```python
from build123d import *

# Parameters (mm, degrees)
SKETCH1_R          = 158.5
BASE_FLANGE1_DEPTH = 1


# Read off the part's stored shape, not the designer's step: Edge-Flange1
# Sheet-metal steps are written as plain solids
with BuildPart() as part:
    # Sketch1 → Base-Flange1 (new body)
    with BuildSketch(Plane(origin=(0, 0, 0), x_dir=(1, 0, 0), z_dir=(0, 1, 0))):
        with Locations(Location((0, 0, 0), (0, 0, 270))):
            Circle(SKETCH1_R)
    extrude(amount=-BASE_FLANGE1_DEPTH)

    # Edge-Flange1 outline → Edge-Flange1 (revolve)
    with BuildSketch(Plane.XY):
        with BuildLine():
            Line((159.2366, -1.7366), (159.2366, -15))
            Line((159.2366, -15), (160.2366, -15))
            Line((160.2366, -15), (160.2366, -1.7366))
            ThreePointArc((160.2366, -1.7366), (159.727961636, -0.508638364), (158.5, 0))
            Line((158.5, 0), (158.5, -1))
            ThreePointArc((158.5, -1), (159.020854855, -1.215745145), (159.2366, -1.7366))
        make_face()
    revolve(axis=Axis((0, 0, 0), (0, 1, 0)))


solid = part.part
```
Design review of the part built by this model. Coordinates are the model's own, in mm. Give positions to 0.01 mm unless a question says otherwise; leave off trailing zeros. Order: outer loops, then holes, each group sorted by start corner. A loop starts at its lowest first (then second) coordinate and runs counter-clockwise, first axis right, second up. Notation, with made-up numbers: M 62.5,59 L 101.5,59 A29 ccw 101.5,83 Z; hole C -18.75,-37 d8. An arc over 180 degrees is marked long. One line per question, with ' | ' between items. Start each with the question number.
Q1. We need section A-A (x = 0). Write out the cut boundary in (y, z), plus the area to 3 significant figures.
Q2. For pin 1 Ø8 at (x, z) = (-110.5, -5) entering from -Y; pin 2 Ø4 at (x, y) = (-70, -12.5) entering from +Z; pin 3 Ø3 at (x, y) = (-14.5, -6.5) entering from +Z, all flat-tipped, find the tip position at first contact; note any pin that passes through.
Q3. The part is to be moulded in two halves that separate along Z. For faces 1 (the face through (152.837, -8.275, -48.131)), 2 (the face through (2, 0, -2)), 3 (the face through (-20.73, -8.46, -157.88)), 4 (the face through (2, -1, -2)), say which applies: +Z half, -Z half, draft (parallel to the pull), parting line (faces both ways), or undercut.
Q4. For L1, parallel to Z at x = 0, y = -5.5; L2, parallel to Y at x = -77, z = 36, list the stretches that pass through material, from the lowest coordinate up. Write a range as [from, to].
Q5. We need section B-B (y = -8.75). Write out the cut boundary in (x, z).
Q6. We need section C-C (z = 0). Write out the cut boundary in (x, y).
Returned:
1) outline: M -15,-160.24 L -1.74,-160.24 A1.74 ccw 0,-158.5 L 0,158.5 A1.74 ccw -1.74,160.24 L -15,160.24 L -15,159.24 L -1.74,159.24 A0.74 cw -1,158.5 L -1,-158.5 A0.74 cw -1.74,-159.24 L -15,-159.24 Z | area: 347 mm2
2) pin 1: y = -1 | pin 2: z = 145.09 | pin 3: z = 159.71
3) face 1: parting line | face 2: draft | face 3: undercut | face 4: undercut
4) L1: [-160.24, -159.24], [159.24, 160.24] | L2: [-1, 0]
5) outline: C 0,0 d320.47; hole C 0,0 d318.47
6) outline: M -160.24,-15 L -159.24,-15 L -159.24,-1.74 A0.74 cw -158.5,-1 L 158.5,-1 A0.74 cw 159.24,-1.74 L 159.24,-15 L 160.24,-15 L 160.24,-1.74 A1.74 ccw 158.5,0 L -158.5,0 A1.74 ccw -160.24,-1.74 Z
